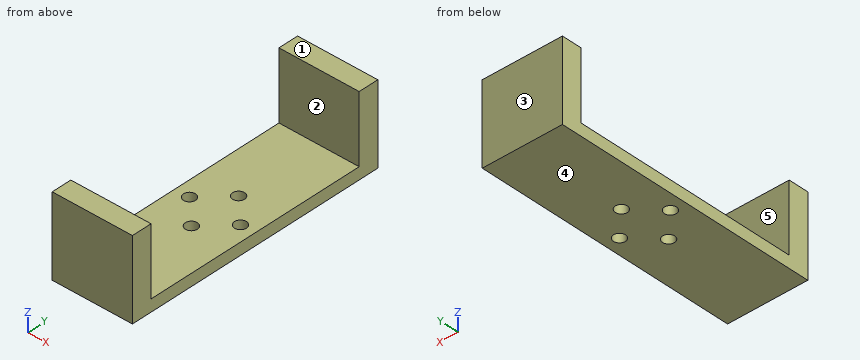
from build123d import *

# Parameters (mm, degrees)
CYLINDER002_R     = 1.5
CYLINDER002_DEPTH = 10
CYLINDER003_R     = 1.5
CYLINDER003_DEPTH = 10
CYLINDER004_R     = 1.5
CYLINDER004_DEPTH = 10
CYLINDER001_R     = 1.5
CYLINDER001_DEPTH = 10
BOX003_W          = 20
BOX003_H          = 65
BOX003_DEPTH      = 3
BOX002_W          = 20
BOX002_H          = 5
BOX002_DEPTH      = 20
BOX001_W          = 20
BOX001_H          = 5
BOX001_DEPTH      = 20


with BuildPart() as h2:
    # Cylinder002 → Cylinder002 (new body)
    with BuildSketch(Plane(origin=(16.35, 32.5, 0), x_dir=(1, 0, 0), z_dir=(0, 0, 1))):
        Circle(CYLINDER002_R)
    extrude(amount=CYLINDER002_DEPTH)


with BuildPart() as h3:
    # Cylinder003 → Cylinder003 (new body)
    with BuildSketch(Plane(origin=(10, 38.85, 0), x_dir=(1, 0, 0), z_dir=(0, 0, 1))):
        Circle(CYLINDER003_R)
    extrude(amount=CYLINDER003_DEPTH)


with BuildPart() as h4:
    # Cylinder004 → Cylinder004 (new body)
    with BuildSketch(Plane(origin=(10, 26.15, 0), x_dir=(1, 0, 0), z_dir=(0, 0, 1))):
        Circle(CYLINDER004_R)
    extrude(amount=CYLINDER004_DEPTH)


with BuildPart() as h1:
    # Cylinder001 → Cylinder001 (new body)
    with BuildSketch(Plane(origin=(3.65, 32.5, 0), x_dir=(1, 0, 0), z_dir=(0, 0, 1))):
        Circle(CYLINDER001_R)
    extrude(amount=CYLINDER001_DEPTH)


with BuildPart() as cut003:
    # Box003 → Box003 (new body)
    with BuildSketch(Plane.XY):
        with Locations((10, 32.5)):
            Rectangle(BOX003_W, BOX003_H)
    extrude(amount=BOX003_DEPTH)

    # Cut: cut H1
    add(h1.part, mode=Mode.SUBTRACT)

    # Cut001: cut H4
    add(h4.part, mode=Mode.SUBTRACT)

    # Cut002: cut H3
    add(h3.part, mode=Mode.SUBTRACT)

    # Cut003: cut H2
    add(h2.part, mode=Mode.SUBTRACT)


with BuildPart() as arm2:
    # Box002 → Box002 (new body)
    with BuildSketch(Plane(origin=(0, 60.5, 0), x_dir=(1, 0, 0), z_dir=(0, 0, 1))):
        with Locations((10, 2.5)):
            Rectangle(BOX002_W, BOX002_H)
    extrude(amount=BOX002_DEPTH)


with BuildPart() as gripper:
    # Box001 → Box001 (new body)
    with BuildSketch(Plane(origin=(0, -0.5, 0), x_dir=(1, 0, 0), z_dir=(0, 0, 1))):
        with Locations((10, 2.5)):
            Rectangle(BOX001_W, BOX001_H)
    extrude(amount=BOX001_DEPTH)

    # Fusion001: union Cut003, Arm2
    add(cut003.part)
    add(arm2.part)


with BuildPart() as gripper_1:
    # Fusion001 placement: moved
    add(gripper.part.moved(Location((11.15, -11.35, 62))))


solid = gripper_1.part
Could you check a few things on this model? Use its own coordinates, in mm. Face numbers are marked on the shaded views. A direction names the side the tool comes from. Give positions to 0.01 mm unless a question says otherwise; leave off trailing zeros. Write each loop counter-clockwise with the first axis right and the second up, starting at its lowest first coordinate (ties: lowest second). Pieces come first, ordered by that corner, then holes. Notation, with made-up numbers: (-34, 28.5) -> (-9, 28.5) arc R21 cw to (-9, 64.5) -> close; hole circle Ø9 at (72.5, 71.25). An arc over 180 degrees is marked (long way). Write each question's results on one line, items separated by ' | '. Start each with the question number.
Q1. We'd pull the mould along Y, two halves only. Please class the marked faces 1, 2 and 3: +Y half, -Y half, draft (parallel to the pull), parting line (faces both ways), or undercut.
Q2. Suppose I cut it at A-A, the plane y = 21.15. List the corners of the cut face in (x, z) for me.
Q3. I need wall thicknesses on probe 1 along X at (y, z) = (21.15, 63.25); probe 2 along Y at (x, z) = (21.15, 63.2). Which ranges of each line are inside material? Lowest first, please.
Q4. Suppose I cut it at B-B, the plane z = 67.5. List the corners of the cut face in (x, y) for me, and give its area (3 significant figures).
Q5. I'm going to push flat-ended pins straight in: pin 1 Ø3 at (y, z) = (-4.5, 67.5) entering from -X; pin 2 Ø4 at (x, y) = (21.15, 27.5) entering from -Z; pin 3 Ø8 at (x, y) = (14, 6.5) entering from +Z. Where does each tip first touch, or does it pass through?
Q6. Suppose I cut it at C-C, the plane x = 14.8. List the corners of the cut face in (y, z) for me, and give its area (3 significant figures).
Q7. Suppose I cut it at D-D, the plane z = 63.5. List the corners of the cut face in (x, y) for me.
Q8. Which directions (+Z, -Z, +X, -X, +Y, -Y) give clear straight access to the entire face, cutting with the end or side of a thin tool? Please do the marked faces 4 and 5.
Outcome:
1) face 1: draft | face 2: undercut | face 3: +Y half
2) outline: (11.15, 62) -> (13.3, 62) -> (13.3, 65) -> (11.15, 65) -> close; (16.3, 62) -> (26, 62) -> (26, 65) -> (16.3, 65) -> close; (29, 62) -> (31.15, 62) -> (31.15, 65) -> (29, 65) -> close
3) probe 1: 11.15 to 13.3, 16.3 to 26, 29 to 31.15 | probe 2: -11.85 to 13.3, 16.3 to 26, 29 to 54.15
4) outline: (11.15, -11.85) -> (31.15, -11.85) -> (31.15, -6.85) -> (11.15, -6.85) -> close; (11.15, 49.15) -> (31.15, 49.15) -> (31.15, 54.15) -> (11.15, 54.15) -> close | area: 200 mm2
5) pin 1: through | pin 2: z = 62 | pin 3: z = 65
6) outline: (-11.85, 62) -> (19.65, 62) -> (19.65, 65) -> (-6.85, 65) -> (-6.85, 82) -> (-11.85, 82) -> close; (22.65, 62) -> (54.15, 62) -> (54.15, 82) -> (49.15, 82) -> (49.15, 65) -> (22.65, 65) -> close | area: 359 mm2
7) outline: (11.15, -11.85) -> (31.15, -11.85) -> (31.15, 54.15) -> (11.15, 54.15) -> close; hole circle Ø3 at (14.8, 21.15); hole circle Ø3 at (21.15, 14.8); hole circle Ø3 at (21.15, 27.5); hole circle Ø3 at (27.5, 21.15)
8) face 4: -Z, +X, -X, +Y, -Y | face 5: +Z, +X, -X
